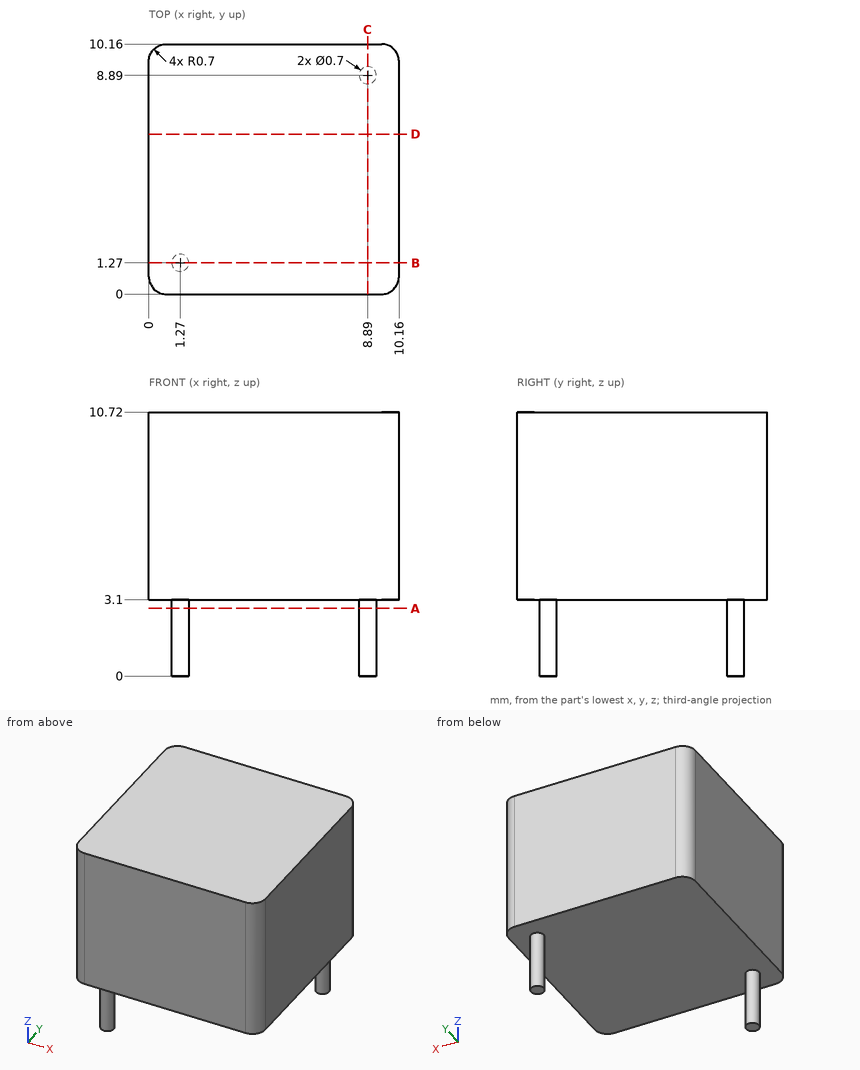
Study the drawing (mm; zero at the part's minimum x, y, z) and answer. Give positions to 0.01 mm unless a question says otherwise; leave off trailing zeros. Order: outer loops, then holes, each group sorted by start corner. A loop starts at its lowest first (then second) coordinate and runs counter-clockwise, first axis right, second up. Notation, with made-up numbers: (-10.75, 8) - (-3.75, 8) arc R19 cw to (-3.75, 26) - close; hole circle Ø1 at (63.5, 21). An arc over 180 degrees is marked (long way). Use one line per item in the form item = value. Start each with the question number.
(1) A cutting plane is placed at B-B, the plane y = 1.27. Write down the section's boundary in (x, z), then the cut area to 3 significant figures.
(2) A cutting plane is placed at A-A, the plane z = 2.75. Write down the section's boundary in (x, y), then the cut area to 3 significant figures.
(3) Flat-ended cylindrical pins translate along their axes: pin 1 Ø3 at (x, z) = (5.5, 8.5) entering from -Y; pin 2 Ø6 at (x, y) = (8, 5) entering from -Z. Find the tip coordinate at first contact, or state that the pin passes through.
(4) A cutting plane is placed at D-D, the plane y = 6.5. Write down the section's boundary in (x, z).
(5) A cutting plane is placed at C-C, the plane x = 8.89. Write down the section's boundary in (y, z), then the cut area to 3 significant figures.
(6) Consider line 1 (Z direction, x = 7.5, y = 6.25); line 2 (X direction, y = 9.5, z = 5.25). Determine where each line is inside the solid, lowest interval first. Write a range as from..to.
Ans:
q1.outline = (0, 3.1) - (0.92, 3.1) - (0.92, 0) - (1.62, 0) - (1.62, 3.1) - (10.16, 3.1) - (10.16, 10.72) - (0, 10.72) - close
q1.area = 79.6 mm^2
q2.outline = circle Ø0.7 at (1.27, 1.27); circle Ø0.7 at (8.89, 8.89)
q2.area = 0.770 mm^2
q3.pin_1 = 0
q3.pin_2 = 3.1
q4.outline = (0, 3.1) - (10.16, 3.1) - (10.16, 10.72) - (0, 10.72) - close
q5.outline = (0, 3.1) - (8.54, 3.1) - (8.54, 0) - (9.24, 0) - (9.24, 3.1) - (10.16, 3.1) - (10.16, 10.72) - (0, 10.72) - close
q5.area = 79.6 mm^2
q6.line_1 = 3.1..10.72
q6.line_2 = 0..10.16
